Could you check a few things on this model? Use its own coordinates, in mm. Coordinates: 2 decimals unless noted, no trailing zeros. Order: outer loops, then holes, each group sorted by start corner. A loop starts at its lowest first (then second) coordinate and runs counter-clockwise, first axis right, second up. Notation, with made-up numbers: (12, 75.25) -> (16, 75.25) arc R22 ccw to (16, 103.25) -> close; hole circle Ø8 at (55.5, -25.75). An arc over 180 degrees is marked (long way). Use a Markdown table: item, result. Add a question column.
1) If we section it at C-C (z = -11): Write out the boundary of the cut face in (x, y), plus the area to 3 significant figures.
2) If I drill on L1, parallel to X at y = 1.75, z = 27.95; L2, parallel to Z at x = 60.5, y = 1.75; L3, parallel to Z at x = 57.5, y = 2.2, over which ranges is the centre line in solid material (lowest first)? Write a range as [from, to].
3) Thinking about a two-plate mould opening in X: for faces 1 (the flat face through (1, 3, -1)), 2 (the cylindrical face through (48.93, 1.48, -47.24)), 3 (the cylindrical face through (-0.664, 1.479, -85.405)), which applies, +X half, -X half, draft (parallel to the pull), parting line (faces both ways), or undercut?
4) If we section it at A-A (x = -3): Write out the boundary of the cut face in (y, z), plus the area to 3 significant figures.
5) If we section it at D-D (x = 20): Write out the boundary of the cut face in (y, z), plus the area to 3 significant figures.
6) If we section it at B-B (y = 0.7): Give the number of separate pieces and of enclosed holes in the cut face, plus the area to 3 significant figures.
7) Will these pins go through, and if not, where does the flat tip stop? pin 1 Ø2.5 at (x, z) = (-50, -88.43) entering from +Y; pin 2 Ø1 at (x, z) = (-50, -100.61) entering from -Y; pin 3 Ø0.9 at (y, z) = (1, -44.5) entering from +X; pin 4 Ø1 at (y, z) = (0.5, 6.5) entering from +X.
```python
from build123d import *

# Parameters (mm, degrees)
SKETCH1_R                                      = 0.79375
SKETCH1_R_2                                    = 1.25
BOSS_EXTRUDE1_DEPTH                            = 3
CSK_FOR_M3_FLAT_HEAD_MACHINE_SCREW1_AT_2_COUNT = 2
CSK_FOR_M3_FLAT_HEAD_MACHINE_SCREW1_AT_2_PITCH = 67.658315793
CSK_FOR_M3_FLAT_HEAD_MACHINE_SCREW1_AT_3_COUNT = 2
CSK_FOR_M3_FLAT_HEAD_MACHINE_SCREW1_AT_3_PITCH = 141.2
CSK_FOR_M3_FLAT_HEAD_MACHINE_SCREW1_AT_4_COUNT = 2
CSK_FOR_M3_FLAT_HEAD_MACHINE_SCREW1_AT_4_PITCH = 156.572946884
CUT_EXTRUDE1_REACH                             = 127.831
SKETCH5_W                                      = 18.5
SKETCH5_H                                      = 10


with BuildPart() as part:
    # Sketch1 → Boss-Extrude1 (new body)
    with BuildSketch(Plane(origin=(0, 0, 0), x_dir=(1, 0, 0), z_dir=(0, 1, 0))):
        with BuildLine():
            ThreePointArc((-43.32807146, 101.968504868), (0, 85.401121174), (43.32807146, 101.968504868))
            ThreePointArc((43.32807146, 101.968504868), (56.388628204, 102.212861373), (58.547766972, 89.329695133))
            ThreePointArc((58.547766972, 89.329695133), (48.991933901, 46.624185339), (67.272511105, 6.8637149))
            ThreePointArc((67.272511105, 6.8637149), (70, 0), (67.272511105, -6.8637149))
            ThreePointArc((67.272511105, -6.8637149), (48.991933901, -46.624185339), (58.547766972, -89.329695133))
            ThreePointArc((58.547766972, -89.329695133), (56.388628204, -102.212861373), (43.32807146, -101.968504868))
            ThreePointArc((43.32807146, -101.968504868), (0, -85.401121174), (-43.32807146, -101.968504868))
            ThreePointArc((-43.32807146, -101.968504868), (-56.388628204, -102.212861373), (-58.547766972, -89.329695133))
            ThreePointArc((-58.547766972, -89.329695133), (-48.991933901, -46.624185339), (-67.272511105, -6.8637149))
            ThreePointArc((-67.272511105, -6.8637149), (-70, 0), (-67.272511105, 6.8637149))
            ThreePointArc((-67.272511105, 6.8637149), (-48.991933901, 46.624185339), (-58.547766972, 89.329695133))
            ThreePointArc((-58.547766972, 89.329695133), (-56.388628204, 102.212861373), (-43.32807146, 101.968504868))
        make_face()
        with Locations(Location((-60, -6.09, 0), (0, 0, 270))):
            Circle(SKETCH1_R, mode=Mode.SUBTRACT)
        with Locations(Location((-50, 88.429654651, 0), (0, 0, 270))):
            Circle(SKETCH1_R, mode=Mode.SUBTRACT)
        with Locations(Location((-50, 100.609654651, 0), (0, 0, 90))):
            Circle(SKETCH1_R, mode=Mode.SUBTRACT)
        with Locations(Location((-60, 6.09, 0), (0, 0, 90))):
            Circle(SKETCH1_R, mode=Mode.SUBTRACT)
        with Locations(Location((60, 6.09, 0), (0, 0, 270))):
            Circle(SKETCH1_R, mode=Mode.SUBTRACT)
        with Locations(Location((60, -6.09, 0), (0, 0, 90))):
            Circle(SKETCH1_R, mode=Mode.SUBTRACT)
        with Locations(Location((50, 88.429654651, 0), (0, 0, 90))):
            Circle(SKETCH1_R, mode=Mode.SUBTRACT)
        with Locations(Location((50, 100.609654651, 0), (0, 0, 270))):
            Circle(SKETCH1_R, mode=Mode.SUBTRACT)
        with Locations(Location((50, -88.429654651, 0), (0, 0, 270))):
            Circle(SKETCH1_R, mode=Mode.SUBTRACT)
        with Locations(Location((50, -100.609654651, 0), (0, 0, 90))):
            Circle(SKETCH1_R, mode=Mode.SUBTRACT)
        with Locations(Location((-50, -88.429654651, 0), (0, 0, 90))):
            Circle(SKETCH1_R, mode=Mode.SUBTRACT)
        with Locations(Location((-50, -100.609654651, 0), (0, 0, 270))):
            Circle(SKETCH1_R, mode=Mode.SUBTRACT)
        with Locations(Location((-34.4, 27.95, 0), (0, 0, 270))):
            Circle(SKETCH1_R_2, mode=Mode.SUBTRACT)
        with Locations(Location((-15.6, 27.95, 0), (0, 0, 270))):
            Circle(SKETCH1_R_2, mode=Mode.SUBTRACT)
        with Locations(Location((-34.4, -27.95, 0), (0, 0, 270))):
            Circle(SKETCH1_R_2, mode=Mode.SUBTRACT)
        with Locations(Location((-15.6, -27.95, 0), (0, 0, 270))):
            Circle(SKETCH1_R_2, mode=Mode.SUBTRACT)
        with Locations(Location((15.6, -27.95, 0), (0, 0, 90))):
            Circle(SKETCH1_R_2, mode=Mode.SUBTRACT)
        with Locations(Location((34.4, -27.95, 0), (0, 0, 90))):
            Circle(SKETCH1_R_2, mode=Mode.SUBTRACT)
        with Locations(Location((15.6, 27.95, 0), (0, 0, 90))):
            Circle(SKETCH1_R_2, mode=Mode.SUBTRACT)
        with Locations(Location((34.4, 27.95, 0), (0, 0, 90))):
            Circle(SKETCH1_R_2, mode=Mode.SUBTRACT)
    extrude(amount=BOSS_EXTRUDE1_DEPTH)

    # Sketch4 → CSK for M3 Flat Head Machine Screw1 (revolve, cut)
    with BuildSketch(Plane(origin=(-33.829157896, 3, -70.836811542), x_dir=(0, 0, 1), z_dir=(1, 0, 0))):
        Polygon((0, 0), (0, 3), (1.7, 3), (1.7, 1.45), (3.15, 0), align=None)
    csk_for_m3_flat_head_machine_screw1 = revolve(axis=Axis((-33.829157896, 9.35, -70.836811542), (0, -1, 0)), mode=Mode.SUBTRACT)

    # CSK for M3 Flat Head Machine Screw1 at 2: CSK for M3 Flat Head Machine Screw1 ×2
    with Locations(*[(i * CSK_FOR_M3_FLAT_HEAD_MACHINE_SCREW1_AT_2_PITCH, 0, 0) for i in range(1, CSK_FOR_M3_FLAT_HEAD_MACHINE_SCREW1_AT_2_COUNT)]):
        add(csk_for_m3_flat_head_machine_screw1, mode=Mode.SUBTRACT)

    # CSK for M3 Flat Head Machine Screw1 at 3: CSK for M3 Flat Head Machine Screw1 ×2
    with Locations(*[(0, 0, i * CSK_FOR_M3_FLAT_HEAD_MACHINE_SCREW1_AT_3_PITCH) for i in range(1, CSK_FOR_M3_FLAT_HEAD_MACHINE_SCREW1_AT_3_COUNT)]):
        add(csk_for_m3_flat_head_machine_screw1, mode=Mode.SUBTRACT)

    # CSK for M3 Flat Head Machine Screw1 at 4: CSK for M3 Flat Head Machine Screw1 ×2
    with Locations(*[Vector(0.4321200893208166, 0, 0.9018160723813751) * (i * CSK_FOR_M3_FLAT_HEAD_MACHINE_SCREW1_AT_4_PITCH) for i in range(1, CSK_FOR_M3_FLAT_HEAD_MACHINE_SCREW1_AT_4_COUNT)]):
        add(csk_for_m3_flat_head_machine_screw1, mode=Mode.SUBTRACT)

    # Sketch5 → Cut-Extrude1 (cut, up to next)
    with BuildSketch(Plane.XZ, mode=Mode.PRIVATE) as cut_extrude1_sk1:
        with Locations((-0.133157896, -44.586811542)):
            Rectangle(SKETCH5_W, SKETCH5_H)
    cut_extrude1_tool1 = extrude(cut_extrude1_sk1.sketch, amount=-CUT_EXTRUDE1_REACH, mode=Mode.PRIVATE) & part.part
    add(cut_extrude1_tool1.solids().sort_by_distance((-0.133158, 0, -44.586812))[0], mode=Mode.SUBTRACT)


solid = part.part
```
Answer sheet:
| question | item | result |
|---|---|---|
| 1 | outline | (-63.67, 0) -> (63.67, 0) -> (63.67, 3) -> (-63.67, 3) -> close |
| 1 | area | 382 mm2 |
| 2 | L1 | [-53.69, -35.65], [-33.15, -16.85], [-14.35, 14.35], [16.85, 33.15], [35.65, 53.69] |
| 2 | L2 | [-15.28, -6.71], [-5.47, 5.47], [6.71, 15.28] |
| 2 | L3 | [-101.13, -87.54], [-20.1, 20.1], [87.54, 101.13] |
| 3 | face 1 | draft |
| 3 | face 2 | +X half |
| 3 | face 3 | undercut |
| 4 | outline | (0, -85.47) -> (3, -85.47) -> (3, -49.59) -> (0, -49.59) -> close; (0, -39.59) -> (3, -39.59) -> (3, 85.47) -> (0, 85.47) -> close |
| 4 | area | 483 mm2 |
| 5 | outline | (0, -88.56) -> (3, -88.56) -> (3, 88.56) -> (0, 88.56) -> close |
| 5 | area | 531 mm2 |
| 6 | separate pieces | 1 |
| 6 | enclosed holes | 25 |
| 6 | area | 20,300 mm2 |
| 7 | pin 1 | y = 3 |
| 7 | pin 2 | through |
| 7 | pin 3 | x = 49.31 |
| 7 | pin 4 | x = 68 |
